Read the model definition and answer for the solid it produces. Units are mm, in the model's axes. Round coordinates to 2 decimals unless told otherwise and drop trailing zeros. Order: outer loops, then holes, each group sorted by start corner. A loop starts at its lowest first (then second) coordinate and runs counter-clockwise, first axis right, second up. Notation, with made-up numbers: (63.5, 38) - (113.5, 38) arc R11 cw to (113.5, 55) - close; hole circle Ø3 at (17.5, 56). An arc over 180 degrees is marked (long way). Answer as a JSON object with one key per item and string values. Group by question number.
Q1. A cutting plane is placed at B-B on z = 11.25. Determine the outline of the cut face in (x, y).
Q2. Consider line 1 (X direction, y = 1.5, z = 11); line 2 (Y direction, x = 6.5, z = 3); line 3 (Z direction, x = 13.5, y = 1.25) (3 decimals). Determine where each line is inside the solid, lowest interval first.
Q3. A cutting plane is placed at A-A on x = 25.4. Count the separate pieces of the cut face and the enclosed holes in it, and give its area (3 significant figures).
Q4. The mould has two halves that part along Z. Classify faces 1 (the cylindrical face through (26.974, 0.402, -1.482)), 2 (the flat face through (-1, 0, 2)), 3 (the flat face through (-15, 1, 6.35)): pulls with the +Z half, pulls with the -Z half, needs draft (parallel to the pull), parting line crosses it, or undercut.
Q5. A cutting plane is placed at C-C on z = -5.25. Determine the outline of the cut face in (x, y).
Q6. Given pin 1 Ø2.5 at (x, z) = (-25.4, -1.275) entering from +Y; pin 2 Ø8 at (x, z) = (12.5, -5) entering from +Y; pin 3 Ø0.8 at (x, y) = (-14.5, 1) entering from +Z; pin 4 Ø1 at (x, y) = (25.5, 2.5) entering from -Z, each flat-ended and moving along its own axis, determine where each tip first touches the part or whether it passes through.
```python
from build123d import *

# Parameters (mm, degrees)
SKETCH1_W                  = 76.2
SKETCH1_H                  = 19.05
BOSS_EXTRUDE1_DEPTH        = 1.5875
SKETCH2_R                  = 3.96875
SKETCH2_R_2                = 2.38125
BOSS_EXTRUDE2_DEPTH        = 76.2
SKETCH4_R                  = 1.5875
CUT_EXTRUDE1_DEPTH         = 41.914713601
CHAMFER1_SIZE              = 0.79375
LPATTERN1_COUNT            = 3
LPATTERN1_PITCH            = 25.4
CHAMFER1_OF_LPATTERN1_SIZE = 0.79375
CUT_EXTRUDE2_START         = -15.24
CUT_EXTRUDE2_DEPTH         = 15.24
LPATTERN2_COUNT            = 5
LPATTERN2_PITCH            = 15.24


with BuildPart() as part:
    # Sketch1 → Boss-Extrude1 (new body)
    with BuildSketch(Plane(origin=(0, 0, 0), x_dir=(1, 0, 0), z_dir=(0, 1, 0))):
        Rectangle(SKETCH1_W, SKETCH1_H)
    extrude(amount=BOSS_EXTRUDE1_DEPTH)

    # Sketch2 → Boss-Extrude2 (add)
    with BuildSketch(Plane(origin=(38.1, 0, 0), x_dir=(0, 0, -1), z_dir=(1, 0, 0))):
        with Locations((-9.525, 3.96875)):
            Circle(SKETCH2_R)
        with Locations((-9.525, 3.96875)):
            Circle(SKETCH2_R_2, mode=Mode.SUBTRACT)
    extrude(amount=-BOSS_EXTRUDE2_DEPTH)

    # Sketch4 → Cut-Extrude1 (cut, through all)
    with BuildSketch(Plane(origin=(0, 1.5875, 0), x_dir=(1, 0, 0), z_dir=(0, 1, 0))):
        with Locations(Location((-25.4, 1.275, 0), (0, 0, 270))):
            Circle(SKETCH4_R)
    cut_extrude1 = extrude(amount=-CUT_EXTRUDE1_DEPTH, mode=Mode.SUBTRACT)

    # Chamfer1
    chamfer1_edges = [part.edges().sort_by_distance(p)[0] for p in [
        (-25.4, 1.5875, -2.8625),
    ]]
    chamfer(chamfer1_edges, length=CHAMFER1_SIZE)

    # LPattern1: Cut-Extrude1 ×3
    with Locations(*[(i * LPATTERN1_PITCH, 0, 0) for i in range(1, LPATTERN1_COUNT)]):
        add(cut_extrude1, mode=Mode.SUBTRACT)

    # Chamfer1 of LPattern1
    chamfer1_of_lpattern1_edges = [part.edges().sort_by_distance(p)[0] for p in [
        (0, 1.5875, -2.8625),
        (25.4, 1.5875, -2.8625),
    ]]
    chamfer(chamfer1_of_lpattern1_edges, length=CHAMFER1_OF_LPATTERN1_SIZE)

    # Sketch5 → Cut-Extrude2 (cut)
    with BuildSketch(Plane(origin=(38.1, 0, 0), x_dir=(0, 0, -1), z_dir=(1, 0, 0)).offset(CUT_EXTRUDE2_START)):
        with BuildLine():
            Line((-6.35, 1.5875), (-6.35, 0))
            Line((-6.35, 0), (-9.525, 0))
            ThreePointArc((-9.525, 0), (-11.299878957, 7.518507914), (-6.35, 1.5875))
        make_face()
    cut_extrude2 = extrude(amount=-CUT_EXTRUDE2_DEPTH, mode=Mode.SUBTRACT)

    # LPattern2: Cut-Extrude2 ×5, 2 skipped
    with Locations(*[(-i * LPATTERN2_PITCH, 0, 0) for i in range(1, LPATTERN2_COUNT) if i not in (1, 3)]):
        add(cut_extrude2, mode=Mode.SUBTRACT)


solid = part.part
```
Result set:
{
 "1": {"outline": "(-38.1, 0.39) - (-22.86, 0.39) - (-22.86, 2.33) - (-38.1, 2.33) - close; (-38.1, 5.61) - (-22.86, 5.61) - (-22.86, 7.54) - (-38.1, 7.54) - close; (-7.62, 0.39) - (7.62, 0.39) - (7.62, 2.33) - (-7.62, 2.33) - close; (-7.62, 5.61) - (7.62, 5.61) - (7.62, 7.54) - (-7.62, 7.54) - close; (22.86, 0.39) - (38.1, 0.39) - (38.1, 2.33) - (22.86, 2.33) - close; (22.86, 5.61) - (38.1, 5.61) - (38.1, 7.54) - (22.86, 7.54) - close"},
 "2": {"line 1": "x = -38.1 to -22.86, -7.62 to 7.62, 22.86 to 38.1", "line 2": "y = 0 to 1.59", "line 3": "z = -9.525 to 6.35"},
 "3": {"separate pieces": "2", "enclosed holes": "1", "area": "52.7 mm²"},
 "4": {"face 1": "undercut", "face 2": "needs draft", "face 3": "pulls with the +Z half"},
 "5": {"outline": "(-38.1, 0) - (38.1, 0) - (38.1, 1.59) - (-38.1, 1.59) - close"},
 "6": {"pin 1": "passes through", "pin 2": "stops at y = 1.59", "pin 3": "stops at z = 6.35", "pin 4": "stops at z = 5.68"}
}
